Autodesk Inventor part; units mm, degrees
ref_plane "YZ Plane" through (0, 0, 0) normal (1, 0, 0) x (0, 1, 0)
ref_plane "XZ Plane" through (0, 0, 0) normal (0, 1, 0) x (-1, 0, 0)
ref_plane "XY Plane" through (0, 0, 0) normal (0, 0, 1) x (1, 0, 0)
sketch "Sketch1" plane through (0, 0, 0) normal (0, 1, 0) x (-1, 0, 0)
  circle A0 centre (0, 0) radius 101.6
  dimension "baseOutsideDiameter" = 203.2
extrude "Extrusion1" add sketch "Sketch1" along normal blind 6.35
sketch "Sketch2" plane through (0, 6.35, 0) normal (0, 1, 0) x (1, 0, 0)
  circle A0 centre (0, 0) radius 101.6
  circle A1 centre (0, 0) radius 95.25
  dimension "d4" = 6.35
  dimension "d5" = 203.2
extrude "Extrusion2" add sketch "Sketch2" along normal blind 50.8
sketch "Sketch3" plane through (0, 6.35, 0) normal (0, 1, 0) x (1, 0, 0)
  circle A0 centre (0, 0) radius 6.35
  dimension "wormDriveDiameer" = 12.7
extrude "Extrusion3" cut sketch "Sketch3" against normal through all
sketch "Sketch5" plane through (0, 6.35, 0) normal (0, 1, 0) x (1, 0, 0)
  circle A0 centre (0, 50.8) radius 12.7
  point P0 (0, 0)
  dimension "wormGearSupportBaseDiameter" = 25.4
  dimension "radiusOfGearSupports" = 50.8
extrude "Extrusion5" add sketch "Sketch5" along normal blind 11.43
pattern_circular "Circular Pattern1" count 6 over 360 about axis through (0, -10, 0) along (0, 1, 0) of "Extrusion5"
sketch "Sketch6" plane through (0, 0, 0) normal (1, 0, 0) x (0, 1, 0)
  arc A0 (36.2401, 78.3957) -> (36.2401, 75.2207) centre (31.75, 76.8082) ccw
  circle A1 centre (31.75, 76.8082) radius 4.7625
  point P0 (0, 0)
extrude "Extrusion6" cut sketch "Sketch6" along normal through all both and the other way through all
equation "\"d4\" = baseThickness"
equation "\"d5\" = baseOutsideDiameter"
properties part number "baseV01"
Geometry check sheet. Reference: the model listing, model coordinates, mm. A direction names the side the tool comes from. Give positions to 0.01 mm unless a question says otherwise; leave off trailing zeros. Order: outer loops, then holes, each group sorted by start corner. A loop starts at its lowest first (then second) coordinate and runs counter-clockwise, first axis right, second up. Notation, with made-up numbers: (-24, 60) - (33, 60) arc R36 cw to (33, 99) - close; hole circle Ø1 at (82.5, -11). An arc over 180 degrees is marked (long way). Answer in a Markdown table with one row per item. Add a question column.
Q1. Mould release check, pull along X, two halves, no side actions. Record for faces 3 (the flat face through (-44, 17.78, 26)), 4 (the flat face through (-44, 17.78, -25)), 5 (the flat face through (-21, 0, 1)): pulls with the +X half, pulls with the -X half, needs draft (parallel to the pull), parting line crosses it, or undercut.
Q2. Tool access check on faces 1 (the cylindrical face through (2.75, 11.98, 63.2)), 2 (the cylindrical face through (-60.567, 27.775, 79.432)). Record the directions out of +Z, -Z, +X, -X, +Y, -Y that give a thin tool (end or side, any length) a straight path to the whole face; none if there is none.
Q3. Cross-section at A-A, the plane z = -25.4. Enter the section's corners in (x, y).
Q4. Cross-section at B-B, the plane y = 31.75. Enter the section's corners in (x, z).
Q5. Material ranges on probe 1 along Z at (x, y) = (0, 35); probe 2 along Y at (x, z) = (32.5, -1), recorded low to high. Write a range as from..to.
Q6. Cross-section at C-C, the plane z = -50.8. Enter the section's corners in (x, y), then the cut area to 3 significant figures.
Q7. Gauge pin test, flat ends, axial feed: pin 1 (10 mm diameter, centred on y = 15, z = -45, fed in from -X); pin 2 (2 mm diameter, centred on y = 9.5, z = -41, fed in from +X); pin 3 (1.5 mm diameter, centred on x = 29, y = 39, fed in from +Z); pin 4 (2 mm diameter, centred on x = 56, z = 34.5, fed in from -Y). Record the tip position at first contact, or that the pin passes through.
Check values:
| question | item | result |
|---|---|---|
| 1 | face 3 | undercut |
| 1 | face 4 | undercut |
| 1 | face 5 | needs draft |
| 2 | face 1 | +Y |
| 2 | face 2 | +X, -X |
| 3 | outline | (-98.37, 0) - (98.37, 0) - (98.37, 57.15) - (91.8, 57.15) - (91.8, 6.35) - (56.69, 6.35) - (56.69, 17.78) - (31.29, 17.78) - (31.29, 6.35) - (-31.29, 6.35) - (-31.29, 17.78) - (-56.69, 17.78) - (-56.69, 6.35) - (-91.8, 6.35) - (-91.8, 57.15) - (-98.37, 57.15) - close |
| 4 | outline | (-71.64, 72.05) arc R101.6 ccw (long way) to (71.64, 72.05) - (62.31, 72.05) arc R95.25 cw (long way) to (-62.31, 72.05) - close; (-60.57, 81.57) - (-49.18, 81.57) arc R95.25 cw to (49.18, 81.57) - (60.57, 81.57) arc R101.6 ccw to start |
| 5 | probe 1 | z = -101.6..-95.25, 95.25..101.6 |
| 5 | probe 2 | y = 0..6.35 |
| 6 | outline | (-87.99, 0) - (87.99, 0) - (87.99, 57.15) - (80.57, 57.15) - (80.57, 6.35) - (12.7, 6.35) - (12.7, 17.78) - (-12.7, 17.78) - (-12.7, 6.35) - (-80.57, 6.35) - (-80.57, 57.15) - (-87.99, 57.15) - close |
| 6 | area | 2,160 mm^2 |
| 7 | pin 1 | stops at x = -93.39 |
| 7 | pin 2 | stops at x = 93.39 |
| 7 | pin 3 | stops at z = 97.59 |
| 7 | pin 4 | stops at y = 0 |
